Autodesk Fusion 360 part; units mm, degrees
sketch "Szkic3" plane through (0, 0, 0) normal (0, 0, 1) x (1, 0, 0)
  line L0 (0, 0) -> (4, 0)
  line L1 (4, 0) -> (4, 10)
  line L2 (4, 10) -> (25, 10)
  line L3 (25, 10) -> (25, 14)
  line L4 (25, 14) -> (0, 14)
  line L5 (0, 14) -> (0, 0)
extrude "Wyciągnięcie proste3" add sketch "Szkic3" along normal blind 55
sketch "Szkic4" plane through (4, 0, 0) normal (1, 0, 0) x (0, 1, 0)
  line L0 (0, 0) -> (10, 0)
  line L1 (10, 0) -> (10, 55)
  line L2 (10, 55) -> (0, 55)
  line L3 (0, 55) -> (0, 0)
  circle A0 centre (6, 9) radius 1.75
  circle A1 centre (6, 47) radius 1.75
  dimension "d19" = 38
  dimension "d20" = 3.5
  dimension "d21" = 3.5
extrude "Wyciągnięcie proste4" cut sketch "Szkic4" against normal blind 4 contours A0 | A1
sketch "Szkic5" plane through (25, 0, 0) normal (1, 0, 0) x (0, 1, 0)
  line L0 (10, 0) -> (14, 0)
  line L1 (14, 0) -> (14, 55)
  line L2 (14, 55) -> (10, 55)
  line L3 (10, 55) -> (10, 0)
  line L4 (14, 55) -> (0, 55)
  line L5 (0, 55) -> (0, 15)
  line L6 (0, 15) -> (14, 15)
  line L7 (14, 15) -> (14, 55)
  line L8 (14, 3) -> (0, 3)
  line L9 (0, 3) -> (0, 0)
  line L10 (0, 0) -> (14, 0)
  line L11 (14, 0) -> (14, 3)
sketch "Szkic6" plane through (0, 14, 0) normal (0, 1, 0) x (-1, 0, 0)
  line L0 (-25, 0) -> (0, 0)
  line L1 (0, 0) -> (0, 55)
  line L2 (0, 55) -> (-25, 55)
  line L3 (-25, 55) -> (-25, 0)
  line L4 (-10, 49) -> (-4, 49)
  line L5 (-4, 49) -> (-4, 29)
  line L6 (-4, 29) -> (-10, 29)
  circle A0 centre (-7, 45) radius 1.8
  line L7 (-5, 20) -> (-15, 20)
  line L8 (-15, 20) -> (-15, 6)
  line L9 (-15, 6) -> (-5, 6)
  line L10 (-5, 6) -> (-5, 20)
  line L11 (-10, 29) -> (-14, 29)
  line L12 (-14, 29) -> (-14, 49)
  line L13 (-14, 49) -> (-10, 49)
  circle A1 centre (-7, 33) radius 1.8
  dimension "d24" = 3.6
  dimension "d25" = 10
  dimension "d26" = 14
  dimension "d27" = 3.6
extrude "Wyciągnięcie proste5" add sketch "Szkic6" along normal blind 6 contours L4 L5 L6 L11 L12 L13 | L7 L8 L9 L10
For this review, take the finished solid that the model builds, in its own axes (mm). A direction names the side the tool comes from. Coordinates: 2 decimals unless noted, no trailing zeros. Write each loop counter-clockwise with the first axis right and the second up, starting at its lowest first coordinate (ties: lowest second). Pieces come first, ordered by that corner, then holes. Notation, with made-up numbers: (23, 75) -> (31, 75) arc R5 ccw to (31, 80) -> close; hole circle Ø5 at (72.5, 78.25). An arc over 180 degrees is marked (long way). Put each result on its own line as item: value.
Q1. Clearance check with flat-ended pins moving along their axes: pin 1 Ø5 at (y, z) = (6, 40.5) entering from +X; pin 2 Ø6.5 at (y, z) = (16, 41) entering from +X; pin 3 Ø10.5 at (x, z) = (14, 26) entering from -Y; pin 4 Ø1.1 at (x, z) = (6.5, 33.5) entering from +Y. State where each tip first meets the part, or that it passes through.
From the geometry:
pin 1: stops at x = 4
pin 2: stops at x = 25
pin 3: stops at y = 10
pin 4: stops at y = 14
Q2. Take a section at C-C, the plane z = 33. State the section outline as (x, y) points.
From the geometry:
outline: (0, 0) -> (4, 0) -> (4, 10) -> (25, 10) -> (25, 14) -> (14, 14) -> (14, 20) -> (8.8, 20) -> (8.8, 14) -> (5.2, 14) -> (5.2, 20) -> (4, 20) -> (4, 14) -> (0, 14) -> close
Q3. Wall thickness on L1, parallel to Z at x = 2.5, y = 6; L2, parallel to Z at x = 7, y = 15.45; L3, parallel to X at y = 8, z = 19: over which ranges is each line inside the solid? List them lowest first.
From the geometry:
L1: z = 0 to 7.25, 10.75 to 45.25, 48.75 to 55
L2: z = 6 to 20, 29 to 31.2, 34.8 to 43.2, 46.8 to 49
L3: x = 0 to 4
Q4. The part is to be moulded in two halves that separate along X. For faces 4 (the cylindrical face through (7.234, 16.958, 31.215)), 5 (the cylindrical face through (2.03, 5.62, 45.29)), 6 (the flat face through (15, 17, 13)), say which applies: +X half, -X half, draft (parallel to the pull), parting line (faces both ways), or undercut.
From the geometry:
face 4: undercut
face 5: draft
face 6: +X half
Q5. Take a section at A-A, the plane y = 15.5. State the section outline as (x, z) points.
From the geometry:
outline: (4, 29) -> (14, 29) -> (14, 49) -> (4, 49) -> close; (5, 6) -> (15, 6) -> (15, 20) -> (5, 20) -> close; hole circle Ø3.6 at (7, 33); hole circle Ø3.6 at (7, 45)
Q6. Tool access review of faces 1 (the flat face through (4, 5, 27)), 2 (the flat face through (9, 17, 49)), 3 (the cylindrical face through (7.234, 16.958, 43.215)): name each direction out of +Z, -Z, +X, -X, +Y, -Y from which nothing blocks a thin tool from reaching the whole face with its end or side.
From the geometry:
face 1: +Z, -Z, +X, -Y
face 2: +Z, +X, -X, +Y
face 3: +Y
Q7. Take a section at D-D, the plane x = 7. State the section outline as (y, z) points.
From the geometry:
outline: (10, 0) -> (14, 0) -> (14, 6) -> (20, 6) -> (20, 20) -> (14, 20) -> (14, 29) -> (20, 29) -> (20, 31.2) -> (14, 31.2) -> (14, 34.8) -> (20, 34.8) -> (20, 43.2) -> (14, 43.2) -> (14, 46.8) -> (20, 46.8) -> (20, 49) -> (14, 49) -> (14, 55) -> (10, 55) -> close
Q8. Take a section at B-B, the plane y = 6. State the section outline as (x, z) points.
From the geometry:
outline: (0, 0) -> (4, 0) -> (4, 7.25) -> (0, 7.25) -> close; (0, 10.75) -> (4, 10.75) -> (4, 45.25) -> (0, 45.25) -> close; (0, 48.75) -> (4, 48.75) -> (4, 55) -> (0, 55) -> close
